Check sheet for the modelled part. Datum: model origin and axes. Units: mm. Face numbers are marked on the shaded views. A direction names the side the tool comes from. Round coordinates to 2 decimals unless told otherwise and drop trailing zeros. Loops run counter-clockwise (first coordinate to the right, second up) from the corner with the lowest first, then second, coordinate; pieces in that order, holes last. Notation, with made-up numbers: (-38.75, -13.5) - (-33.75, -13.5) arc R30 ccw to (-33.75, 21.5) - close; hole circle Ø1 at (6, -1). An arc over 180 degrees is marked (long way). Return JSON: item names as keys, results as strings.
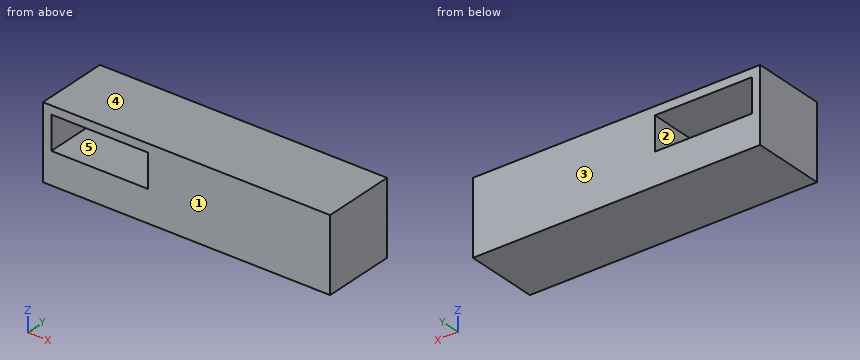
from build123d import *

# Parameters (mm, degrees)
F0_W     = 172
F0_H     = 44
F0_W_2   = 58
F0_H_2   = 20
F1_DEPTH = 22


with BuildPart() as f1:
    # F0 (on Front) → F1 (new body, symmetric)
    with BuildSketch(Plane.XZ):
        Rectangle(F0_W, F0_H)
        with Locations((-52, 7)):
            Rectangle(F0_W_2, F0_H_2, mode=Mode.SUBTRACT)
    extrude(amount=F1_DEPTH, both=True)


solid = f1.part
Q1. Sectioned sample at C-C (z = -1.5). Enter the section's corners in (x, y).
Answer key:
{"outline": "(-86, -22) - (-81, -22) - (-81, 22) - (-86, 22) - close; (-23, -22) - (86, -22) - (86, 22) - (-23, 22) - close"}
Q2. Tool access check on the marked faces 1 and 2. Record the directions out of +Z, -Z, +X, -X, +Y, -Y that give a thin tool (end or side, any length) a straight path to the whole face; none if there is none.
Answer key:
{"face 1": "+Z, -Z, +X, -X, -Y", "face 2": "+Y, -Y"}
Q3. Scan lines: probe 1 along X at (y, z) = (-14.5, 16.5); probe 2 along Z at (x, y) = (-56.5, 10). Record each from-to range of solid material in increasing order. Write a range as [from, to].
Answer key:
{"probe 1": "x = [-86, -81], [-23, 86]", "probe 2": "z = [-22, -3], [17, 22]"}
Q4. Sectioned sample at B-B (x = -31.5). Enter the section's corners in (y, z).
Answer key:
{"outline": "(-22, -22) - (22, -22) - (22, -3) - (-22, -3) - close; (-22, 17) - (22, 17) - (22, 22) - (-22, 22) - close"}
Q5. Draft check along Z on the marked faces 3, 4 and 5. Enter one of: released by +Z, released by -Z, zero draft, split by the parting line, or undercut.
Answer key:
{"face 3": "zero draft", "face 4": "released by +Z", "face 5": "undercut"}
Q6. Sectioned sample at A-A (y = 7.5). Enter the section's corners in (x, z), plus the area to 3 significant figures.
Answer key:
{"outline": "(-86, -22) - (86, -22) - (86, 22) - (-86, 22) - close; hole (-81, -3) - (-23, -3) - (-23, 17) - (-81, 17) - close", "area": "6,410 mm²"}
